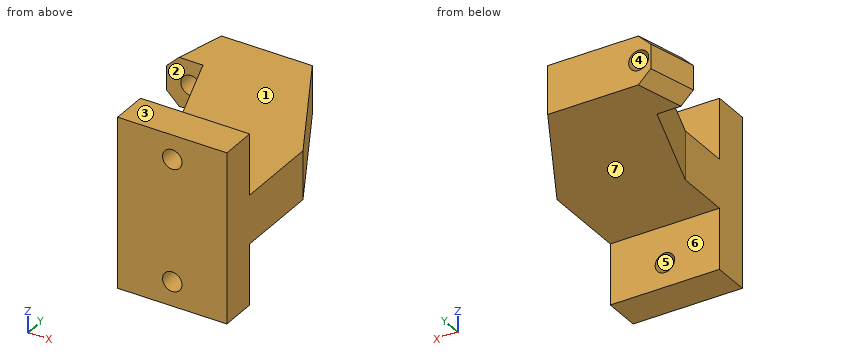
```python
from build123d import *

# Parameters (mm, degrees)
F1_DEPTH  = 8
F2_W      = 18
F2_H      = 6
F3_DEPTH  = 10
F4_W      = 18
F4_H      = 6
F5_DEPTH  = 10
F6_SIZE   = 2
F7_SIZE   = 2
F8_R      = 1.65
F9_DEPTH  = 25
F10_R     = 1.6
F11_DEPTH = 25


with BuildPart() as f1:
    # F0 (on Top) → F1 (new body)
    with BuildSketch(Plane.XY):
        Polygon((-17.884355, 24.999997), (-19.884355, 16.999997), (-13.884355, 16.999997), (-7.884355, 0), (-7.884355, -15.000003), (10.115645, -15.000003), (10.115645, 4.999997), (-0.884355, 24.999997), align=None)
    extrude(amount=F1_DEPTH)

    # F2 (on face) → F3 (join)
    with BuildSketch(Plane.XY.offset(8)):
        with Locations((1.115645, -12.000003)):
            Rectangle(F2_W, F2_H)
    extrude(amount=F3_DEPTH)

    # F4 (on face) → F5 (join)
    with BuildSketch(Plane(origin=(0, 0, 0), x_dir=(1, 0, 0), z_dir=(0, 0, -1))):
        with Locations((1.115645, 12.000003)):
            Rectangle(F4_W, F4_H)
    extrude(amount=F5_DEPTH)

    # F6
    f6_edges = [f1.edges().sort_by_distance(p)[0] for p in [
        (-18.884355, 20.999997, 0),
    ]]
    chamfer(f6_edges, length=F6_SIZE)

    # F7
    f7_edges = [f1.edges().sort_by_distance(p)[0] for p in [
        (-18.884355, 20.999997, 8),
    ]]
    chamfer(f7_edges, length=F7_SIZE)

    # F8 (on face) → F9 (cut)
    with BuildSketch(Plane(origin=(0, 24.999997, 0), x_dir=(-1, 0, 0), z_dir=(0, 1, 0))):
        with Locations((15.884355, 4)):
            Circle(F8_R)
    extrude(amount=-F9_DEPTH, mode=Mode.SUBTRACT)

    # F10 (on face) → F11 (cut)
    with BuildSketch(Plane.XZ.offset(15.000003)):
        with Locations((1.115645, 14)):
            Circle(F10_R)
        with Locations((1.115645, -6)):
            Circle(F10_R)
    extrude(amount=-F11_DEPTH, mode=Mode.SUBTRACT)


solid = f1.part
```
Read the model definition and answer for the solid it produces. Units are mm, in the model's axes. Face numbers are marked on the shaded views. A direction names the side the tool comes from. Round coordinates to 2 decimals unless told otherwise and drop trailing zeros. Loops run counter-clockwise (first coordinate to the right, second up) from the corner with the lowest first, then second, coordinate; pieces in that order, holes last. Notation, with made-up numbers: (26.5, 16.25) -> (84.5, 16.25) arc R18 ccw to (84.5, 28.25) -> close; hole circle Ø1 at (22, 63). An arc over 180 degrees is marked (long way). One line per item, written item: value.
1) A cutting plane is placed at A-A (z = 14). Determine the outline of the cut face in (x, y).
Answer list:
outline: (-7.88, -15) -> (-0.48, -15) -> (-0.48, -9) -> (-7.88, -9) -> close; (2.72, -15) -> (10.12, -15) -> (10.12, -9) -> (2.72, -9) -> close
2) For the marked faces 1, 2 and 3, determine the directions among +Z, -Z, +X, -X, +Y, -Y from which every point of the face is accessible in a straight line to the end or side of a thin tool.
Answer list:
face 1: +Z, +X, -X, +Y
face 2: +Z, -Z, -X, -Y
face 3: +Z, +X, -X, +Y, -Y
3) A cutting plane is placed at D-D (z = 4). Determine the outline of the cut face in (x, y).
Answer list:
outline: (-19.88, 17) -> (-17.53, 17) -> (-17.53, 25) -> (-17.88, 25) -> close; (-14.23, 17) -> (-13.88, 17) -> (-7.88, 0) -> (-7.88, -15) -> (10.12, -15) -> (10.12, 5) -> (-0.88, 25) -> (-14.23, 25) -> close
4) Consider L1, parallel to Y at x = -17.5, z = 4.5; L2, parallel to Z at x = 3.75, y = 16.5; L3, parallel to Y at x = -4.25, z = -5. Determine where each line is inside the solid, lowest interval first. Write a range as [from, to].
Answer list:
L1: y = [17, 25]
L2: z = [0, 8]
L3: y = [-15, -9]
5) A cutting plane is placed at C-C (y = -11). Determine the outline of the cut face in (x, z), and give its area (3 significant figures).
Answer list:
outline: (-7.88, -10) -> (10.12, -10) -> (10.12, 18) -> (-7.88, 18) -> close; hole circle Ø3.2 at (1.12, -6); hole circle Ø3.2 at (1.12, 14)
area: 488 mm²
6) The mould has two halves that part along Z. Classify the marked faces 4, 5, 6 and 7: pulls with the +Z half, pulls with the -Z half, needs draft (parallel to the pull), parting line crosses it, or undercut.
Answer list:
face 4: undercut
face 5: undercut
face 6: needs draft
face 7: pulls with the -Z half
7) Flat-ended cylindrical pins translate along their axes: P1, Ø1, axis at x = 0.5, y = 14.5, coming from the +Z side; P2, Ø3, axis at x = -16.5, z = 4.5, coming from the -Y side; P3, Ø4, axis at x = 0, z = 12.5, coming from the +Y side. Find the tip coordinate at first contact, or state that the pin passes through.
Answer list:
P1: stops at z = 8
P2: stops at y = 17
P3: stops at y = -9
8) A cutting plane is placed at B-B (x = 1). Determine the outline of the cut face in (y, z), and give its area (3 significant figures).
Answer list:
outline: (-15, -10) -> (-9, -10) -> (-9, -7.6) -> (-15, -7.6) -> close; (-15, -4.4) -> (-9, -4.4) -> (-9, 0) -> (21.57, 0) -> (21.57, 8) -> (-9, 8) -> (-9, 12.4) -> (-15, 12.4) -> close; (-15, 15.6) -> (-9, 15.6) -> (-9, 18) -> (-15, 18) -> close
area: 374 mm²
